Source: CAD feature listing. Evaluate the final solid. Frame: model axes, mm. Face numbers are marked on the shaded views. Give positions to 0.01 mm unless a question says otherwise; leave off trailing zeros. Order: outer loops, then holes, each group sorted by start corner. A loop starts at its lowest first (then second) coordinate and runs counter-clockwise, first axis right, second up. Notation, with made-up numbers: (0.25, 66) -> (47.25, 66) arc R15 ccw to (47.25, 80) -> close; hole circle Ø6 at (82.25, -27). An arc over 180 degrees is marked (long way). Answer in a Markdown table with one row per item.
```python
from build123d import *

# Parameters (mm, degrees)
F0_R     = 11.5
F1_DEPTH = 15
F3_D     = 4.2
F4_D     = 10.3
F5_R     = 6
F6_DEPTH = 4.2


with BuildPart() as f1:
    # F0 (on Front) → F1 (new body)
    with BuildSketch(Plane.XZ):
        with BuildLine():
            Line((71.156512348, 11.0983319967), (0, 20))
            Line((0, 20), (-51.8216221637, 12.3665554094))
            ThreePointArc((-51.8216221637, 12.3665554094), (-62.5, 0), (-51.8216221637, -12.3665554094))
            Line((-51.8216221637, -12.3665554094), (0, -20))
            Line((0, -20), (90.6974930025, -3.9387185113))
            ThreePointArc((90.6974930025, -3.9387185113), (93.9850344054, -0.3456888592), (91.3653125965, 3.7597767904))
            Line((91.3653125965, 3.7597767904), (71.156512348, 11.0983319967))
        make_face()
        Circle(F0_R, mode=Mode.SUBTRACT)
    extrude(amount=F1_DEPTH)

    # F3 (through all)
    with Locations(Plane(origin=(0, 0, 0), x_dir=(-1, 0, 0), z_dir=(0, 1, 0))):
        with Locations((-60, 0), (-45, 0)):
            Hole(F3_D / 2)

    # F4 (through all)
    with Locations(Plane(origin=(0, 0, 0), x_dir=(1, 0, 0), z_dir=(0, 1, 0))):
        with Locations((-50, 0)):
            Hole(F4_D / 2)

    # F5 (on face) → F6 (cut)
    with BuildSketch(Plane(origin=(11.8507540815, 0, 32.6344239833), x_dir=(0.9399441976, 0, -0.3413281491), z_dir=(0.3413281491, 0, 0.9399441976))):
        with Locations((73.8449777845, -7.5)):
            Circle(F5_R)
    extrude(amount=-F6_DEPTH, mode=Mode.SUBTRACT)


solid = f1.part
```
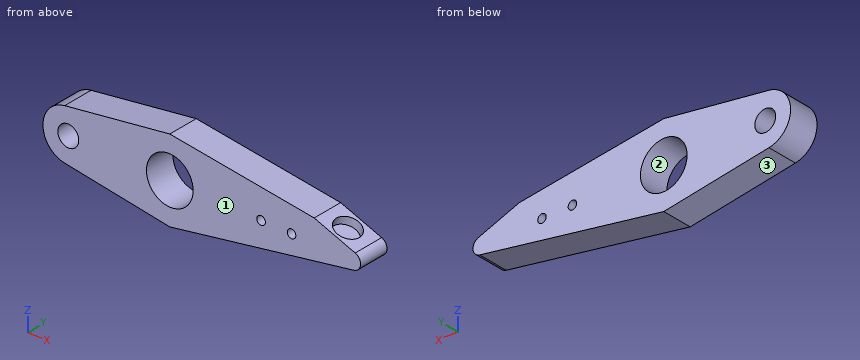
(1) Section query A-A (x = 45). Return the cut outline in (y, z).
A:
| item | result |
|---|---|
| outline | (-15, -12.03) -> (0, -12.03) -> (0, -2.1) -> (-15, -2.1) -> close; (-15, 2.1) -> (0, 2.1) -> (0, 14.37) -> (-15, 14.37) -> close |
(2) First-contact query: pin 1 Ø2 at (x, y) = (45.5, -2.5) entering from +Z; pin 2 Ø2 at (y, z) = (-3, 3.5) entering from -X; pin 3 Ø9.5 at (x, z) = (-50, 0) entering from +Y; pin 4 Ø1.5 at (x, y) = (65.5, -3) entering from -Z. Flat tips, straight axial feed; report the tip coordinate or a pass-through.
A:
| item | result |
|---|---|
| pin 1 | stops at z = 14.43 |
| pin 2 | stops at x = -62.25 |
| pin 3 | passes through |
| pin 4 | stops at z = -8.53 |
(3) Section query C-C (x = -50). Return the cut outline in (y, z), plus the area to 3 significant figures.
A:
| item | result |
|---|---|
| outline | (-15, -12.63) -> (0, -12.63) -> (0, -5.15) -> (-15, -5.15) -> close; (-15, 5.15) -> (0, 5.15) -> (0, 12.63) -> (-15, 12.63) -> close |
| area | 225 mm^2 |
(4) Section query B-B (y = -10.25). Return the cut outline in (x, z).
A:
| item | result |
|---|---|
| outline | (-51.82, -12.37) -> (0, -20) -> (90.7, -3.94) arc R4 ccw to (91.37, 3.76) -> (86.27, 5.61) -> (84.84, 1.66) -> (74.81, 5.3) -> (76.25, 9.25) -> (71.16, 11.1) -> (0, 20) -> (-51.82, 12.37) arc R12.5 ccw to start; hole circle Ø10.3 at (-50, 0); hole circle Ø23 at (0, 0); hole circle Ø4.2 at (45, 0); hole circle Ø4.2 at (60, 0) |
(5) Section query D-D (y = -3.5). Return the cut outline in (x, z).
A:
| item | result |
|---|---|
| outline | (-51.82, -12.37) -> (0, -20) -> (90.7, -3.94) arc R4 ccw to (91.37, 3.76) -> (85.46, 5.9) -> (84.03, 1.95) -> (75.62, 5.01) -> (77.06, 8.96) -> (71.16, 11.1) -> (0, 20) -> (-51.82, 12.37) arc R12.5 ccw to start; hole circle Ø10.3 at (-50, 0); hole circle Ø23 at (0, 0); hole circle Ø4.2 at (45, 0); hole circle Ø4.2 at (60, 0) |
(6) Ray query, probe 1 along Z at (x, y) = (0, -9.75); probe 2 along Z at (x, y) = (-50, -9.75); probe 3 along X at (y, z) = (-4.75, 8). Return the intervals inside material, ascending.
A:
| item | result |
|---|---|
| probe 1 | z = -20 to -11.5, 11.5 to 20 |
| probe 2 | z = -12.63 to -5.15, 5.15 to 12.63 |
| probe 3 | x = -59.6 to -8.26, 8.26 to 75.79 |
(7) Pull-direction query (Z, two-part tool) for the marked faces 1, 2 and 3; classes: +Z half, -Z half, draft (parallel to the pull), parting line (faces both ways), or undercut.
A:
| item | result |
|---|---|
| face 1 | draft |
| face 2 | undercut |
| face 3 | -Z half |
